Part model, mm, in its own coordinate system. A direction names the side the tool comes from. Round coordinates to 2 decimals unless told otherwise and drop trailing zeros. Loops run counter-clockwise (first coordinate to the right, second up) from the corner with the lowest first, then second, coordinate; pieces in that order, holes last. Notation, with made-up numbers: (46.5, 3) -> (85.5, 3) arc R20 ccw to (85.5, 27) -> close; hole circle Ø5 at (-7.75, -0.75). An arc over 180 degrees is marked (long way). Answer as CSV lines item,"result".
from build123d import *

# Parameters (mm, degrees)
SKETCH1_W                      = 61.6458
SKETCH1_H                      = 61.6458
BOSS_EXTRUDE1_DEPTH            = 3.175
F_3_16_0_1875_DIAMETER_HOLE1_D = 4.7625
F_8_CLEARANCE_HOLE1_D          = 4.4958
F_10_CLEARANCE_HOLE2_D         = 5.1054
FILLET1_R                      = 4.4958
SKETCH9_R                      = 28.452559636
CUT_EXTRUDE2_DEPTH             = 4.175
SKETCH9_4_R                    = 18.465762264
CUT_EXTRUDE3_DEPTH             = 4.175
FILLET3_R                      = 4.4958


with BuildPart() as part:
    # Sketch1 → Boss-Extrude1 (new body)
    with BuildSketch(Plane.XY):
        Rectangle(SKETCH1_W, SKETCH1_H)
    extrude(amount=BOSS_EXTRUDE1_DEPTH)

    # 3/16 (0.1875) Diameter Hole1 (through all)
    with Locations(Plane.XY.offset(3.175)):
        with Locations((0, -14.685), (0, 14.685)):
            Hole(F_3_16_0_1875_DIAMETER_HOLE1_D / 2)

    # #8 Clearance Hole1 (through all)
    with Locations(Plane.XY.offset(3.175)):
        with Locations((-25.4, 25.4), (-25.4, -25.4), (25.4, -25.4), (25.4, 25.4)):
            Hole(F_8_CLEARANCE_HOLE1_D / 2)

    # #10 Clearance Hole2 (through all)
    with Locations(Plane.XY.offset(3.175)):
        with Locations((0, 0)):
            Hole(F_10_CLEARANCE_HOLE2_D / 2)

    # Fillet1
    fillet1_edges = [part.edges().sort_by_distance(p)[0] for p in [
        (-30.8229, 30.8229, 1.5875),
        (30.8229, 30.8229, 1.5875),
        (30.8229, -30.8229, 1.5875),
        (-30.8229, -30.8229, 1.5875),
    ]]
    fillet(fillet1_edges, radius=FILLET1_R)

    # Sketch9 → Cut-Extrude2 (cut, through all)
    with BuildSketch(Plane.XY.offset(3.175)):
        with Locations((0, 50.147959636)):
            Circle(SKETCH9_R)
    cut_extrude2 = extrude(amount=-CUT_EXTRUDE2_DEPTH, mode=Mode.SUBTRACT)

    # Sketch9<4> → Cut-Extrude3 (cut, through all)
    with BuildSketch(Plane.XY.offset(3.175)):
        with Locations((27.368462264, 0)):
            Circle(SKETCH9_4_R)
    cut_extrude3 = extrude(amount=-CUT_EXTRUDE3_DEPTH, mode=Mode.SUBTRACT)

    # Mirror1: Cut-Extrude2 across plane
    add(cut_extrude2.mirror(Plane.ZX), mode=Mode.SUBTRACT)

    # Mirror2: Cut-Extrude3 across plane
    add(cut_extrude3.mirror(Plane(origin=(0, 0, 0), x_dir=(0, 0, 1), z_dir=(1, 0, 0))), mode=Mode.SUBTRACT)

    # Fillet3
    fillet3_edges = [part.edges().sort_by_distance(p)[0] for p in [
        (-30.8229, 18.139769456, 1.5875),
        (-30.8229, -18.139769456, 1.5875),
        (20.882773281, 30.8229, 1.5875),
        (-20.882773281, 30.8229, 1.5875),
        (30.8229, -18.139769456, 1.5875),
        (30.8229, 18.139769456, 1.5875),
        (-20.882773281, -30.8229, 1.5875),
        (20.882773281, -30.8229, 1.5875),
    ]]
    fillet(fillet3_edges, radius=FILLET3_R)


solid = part.part
Q1. Saw through at D-D, the plane y = -25.4. Write the cut outline in (x, z) (3 decimals).
Geometry results:
outline,"(-30.823, 0) -> (-27.648, 0) -> (-27.648, 3.175) -> (-30.823, 3.175) -> close; (-23.152, 0) -> (-14.039, 0) -> (-14.039, 3.175) -> (-23.152, 3.175) -> close; (14.039, 0) -> (23.152, 0) -> (23.152, 3.175) -> (14.039, 3.175) -> close; (27.648, 0) -> (30.823, 0) -> (30.823, 3.175) -> (27.648, 3.175) -> close"
Q2. Saw through at B-B, the plane x = 0. Write the cut outline in (y, z) (3 decimals), then the cut area to 3 significant figures.
Geometry results:
outline,"(-21.695, 0) -> (-17.066, 0) -> (-17.066, 3.175) -> (-21.695, 3.175) -> close; (-12.304, 0) -> (-2.553, 0) -> (-2.553, 3.175) -> (-12.304, 3.175) -> close; (2.553, 0) -> (12.304, 0) -> (12.304, 3.175) -> (2.553, 3.175) -> close; (17.066, 0) -> (21.695, 0) -> (21.695, 3.175) -> (17.066, 3.175) -> close"
area,"91.3 mm2"
Q3. Saw through at A-A, the plane y = 0. Write the cut outline in (x, z) (3 decimals), then the cut area to 3 significant figures.
Geometry results:
outline,"(-8.903, 0) -> (-2.553, 0) -> (-2.553, 3.175) -> (-8.903, 3.175) -> close; (2.553, 0) -> (8.903, 0) -> (8.903, 3.175) -> (2.553, 3.175) -> close"
area,"40.3 mm2"
Q4. Drill centre lines: line 1 along Y through (x, z) = (0, 1.6); line 2 along X through (y, z) = (-25, 1.4); line 3 along Y through (x, z) = (26, 2). Where is each one in solid material? Low to high.
Geometry results:
line 1,"-21.7 to -17.07, -12.3 to -2.55, 2.55 to 12.3, 17.07 to 21.7"
line 2,"-30.82 to -27.61, -23.19 to -13.31, 13.31 to 23.19, 27.61 to 30.82"
line 3,"-30.82 to -27.57, -23.23 to -18.41, 18.41 to 23.23, 27.57 to 30.82"
Q5. Two-plate mould, pull along X, no slides. Class faces 1 (the face through (-7, 0, 0)), 2 (the face through (21.07, 30.49, 1.61)), 3 (the face through (29.47, -29.54, 1.61)): pulls with the +X half, pulls with the -X half, needs draft (parallel to the pull), parting line crosses it, or undercut.
Geometry results:
face 1,"needs draft"
face 2,"undercut"
face 3,"pulls with the +X half"
Q6. Saw through at C-C, the plane z = 0.8. Give the number of separate pieces and of enclosed holes in the cut face, then the cut area to 3 significant figures.
Geometry results:
separate pieces,"1"
enclosed holes,"7"
area,"1,790 mm2"
Q7. Which spindle directions (+Z, -Z, +X, -X, +Y, -Y) get a long thin tool onto all of the face, cutting with end or side? Do faces 4 (the face through (25.887, 23.206, 1.565)), 5 (the face through (29.61, 19.867, 1.61)), 6 (the face through (-25, 30.823, 2)), 7 (the face through (-21.07, -30.49, 1.61)), 8 (the face through (-21.11, 30.51, 1.61)). Say none if no direction does.
Geometry results:
face 4,"+Z, -Z"
face 5,"+Z, -Z, +X"
face 6,"+Z, -Z, +X, -X, +Y"
face 7,"+Z, -Z, -Y"
face 8,"+Z, -Z, +Y"
Q8. Drop flat-ended pins along their axis: P1, Ø6.5, axis at x = 0, y = 0, coming from the +Z side (3 decimals); P2, Ø1, axis at y = -12.5, z = 2.5, coming from the +X side; P3, Ø1, axis at y = 15, z = 1, coming from the +X side. Give the stop position or say it passes through.
Geometry results:
P1,"z = 3.175"
P2,"x = 14.25"
P3,"x = 17.33"
